Design review of the part built by this model. Coordinates are the model's own, in mm. A direction names the side the tool comes from. Coordinates: 2 decimals unless noted, no trailing zeros. Order: outer loops, then holes, each group sorted by start corner. A loop starts at its lowest first (then second) coordinate and runs counter-clockwise, first axis right, second up. Notation, with made-up numbers: (-9.75, 67.5) - (4.25, 67.5) arc R27 cw to (4.25, 104.5) - close; hole circle Ø1 at (-36.75, 42). An arc over 180 degrees is marked (long way). Write each question's results on one line, items separated by ' | '. Start each with the question number.
```python
from build123d import *
from OCP.BRepFilletAPI import BRepFilletAPI_MakeChamfer

# Parameters (mm, degrees)
BOSS_EXTRUDE1_DEPTH = 76.2
BOSS_EXTRUDE3_DEPTH = 152.4
SKETCH2_W           = 134.62
SKETCH2_H           = 39.37
CUT_EXTRUDE1_DEPTH  = 94.414090077
CHAMFER1_SIZE       = 2.54
SKETCH5_W           = 7.62
SKETCH5_H           = 6.35
BOSS_EXTRUDE4_DEPTH = 8.89
SKETCH6_W           = 134.62
SKETCH6_H           = 7.62
CUT_EXTRUDE2_DEPTH  = 95.091487925
FILLET1_R           = 2.54
FILLET2_R           = 1.27
CHAMFER2_SIZE       = 1.651
CHAMFER2_SIZE2      = 2.963635699


with BuildPart() as part:
    # Sketch1 → Boss-Extrude1 (new, symmetric)
    with BuildSketch(Plane(origin=(0, 0, 0), x_dir=(0, 0, -1), z_dir=(1, 0, 0))):
        Polygon((0, 0), (0, 12.7), (-9.525, 12.7), (-9.525, -50.8), (8.89, -50.8), (8.89, 0), align=None)
    extrude(amount=BOSS_EXTRUDE1_DEPTH, both=True)

    # Sketch4 → Boss-Extrude3 (add)
    with BuildSketch(Plane(origin=(76.2, 0, 0), x_dir=(0, 0, -1), z_dir=(1, 0, 0))):
        Polygon((8.89, 0), (21.59, 0), (21.59, -6.35), (8.89, -11.43), align=None)
    extrude(amount=-BOSS_EXTRUDE3_DEPTH)

    # Sketch2 → Cut-Extrude1 (cut, through all)
    with BuildSketch(Plane(origin=(0, 0, -8.89), x_dir=(-1, 0, 0), z_dir=(0, 0, -1))):
        with Locations((0, -31.115)):
            Rectangle(SKETCH2_W, SKETCH2_H)
    extrude(amount=-CUT_EXTRUDE1_DEPTH, mode=Mode.SUBTRACT)

    # Chamfer1
    chamfer1_edges = [part.edges().sort_by_distance(p)[0] for p in [
        (76.2, 12.7, 4.7625),
        (-76.2, 12.7, 4.7625),
    ]]
    chamfer(chamfer1_edges, length=CHAMFER1_SIZE)

    # Sketch5 → Boss-Extrude4 (add)
    with BuildSketch(Plane(origin=(76.2, 0, 0), x_dir=(0, 0, -1), z_dir=(1, 0, 0))):
        with Locations((17.78, 3.175)):
            Rectangle(SKETCH5_W, SKETCH5_H)
    boss_extrude4 = extrude(amount=-BOSS_EXTRUDE4_DEPTH)

    # Mirror1: Boss-Extrude4 across plane
    add(boss_extrude4.mirror(Plane(origin=(0, 0, 0), x_dir=(0, 0, 1), z_dir=(1, 0, 0))))

    # Sketch6 → Cut-Extrude2 (cut, through all)
    with BuildSketch(Plane(origin=(0, 0, 0), x_dir=(1, 0, 0), z_dir=(0, 1, 0))):
        with Locations((0, 17.78)):
            Rectangle(SKETCH6_W, SKETCH6_H)
    extrude(amount=-CUT_EXTRUDE2_DEPTH, mode=Mode.SUBTRACT)

    # Fillet1
    fillet1_edges = [part.edges().sort_by_distance(p)[0] for p in [
        (-71.755, -11.43, -8.89),
        (71.755, -11.43, -8.89),
        (-67.31, -4.699, -13.97),
        (67.31, -4.699, -13.97),
    ]]
    fillet(fillet1_edges, radius=FILLET1_R)

    # Fillet2
    fillet2_edges = [part.edges().sort_by_distance(p)[0] for p in [
        (67.31, 0, -15.24),
        (-67.31, 0, -15.24),
        (71.755, 0, -13.97),
        (-71.755, 0, -13.97),
    ]]
    fillet(fillet2_edges, radius=FILLET2_R)

    # Chamfer2: one chamfer whose edges measure the first distance from different faces: ONE call of the kernel's chamfer builder (chamfer() names one face for all edges)
    chamfer2_edges_1 = [part.edges().sort_by_distance(p)[0] for p in [
        (-71.755, -6.35, -21.59),
    ]]
    chamfer2_side_1 = [part.faces().sort_by_distance(p)[0] for p in [
        (-71.755, 0, -21.59),
    ]]
    chamfer2_edges_2 = [part.edges().sort_by_distance(p)[0] for p in [
        (71.755, 6.35, -21.59),
        (-71.755, 6.35, -21.59),
    ]]
    chamfer2_edges_3 = [part.edges().sort_by_distance(p)[0] for p in [
        (71.755, -6.35, -21.59),
    ]]
    chamfer2_side_3 = [part.faces().sort_by_distance(p)[0] for p in [
        (71.755, 0, -21.59),
    ]]
    chamfer2 = BRepFilletAPI_MakeChamfer(part.part.solid().wrapped)
    for e in chamfer2_edges_1:
        chamfer2.Add(CHAMFER2_SIZE, CHAMFER2_SIZE2, e.wrapped, chamfer2_side_1[0].wrapped)  # the first distance lies on this face
    for e in chamfer2_edges_2:
        chamfer2.Add(CHAMFER2_SIZE, e.wrapped)
    for e in chamfer2_edges_3:
        chamfer2.Add(CHAMFER2_SIZE, CHAMFER2_SIZE2, e.wrapped, chamfer2_side_3[0].wrapped)  # the first distance lies on this face
    add(Compound.cast(chamfer2.Shape()), mode=Mode.REPLACE)


solid = part.part
```
(1) Take a section at A-A (y = -43). State the section outline as (x, z) points (3 decimals), plus the area to 3 significant figures.
(2) To check wall thickness, follow line 1 along X through (y, z) = (-25, -8); line 2 along Z through (x, y) = (69, -40) (3 decimals); line 3 along Z through (x, y) = (-28, -4.5) (3 decimals). State the ranges of each line that lie inside material, in increasing order. Write a range as [from, to].
(3) Take a section at C-C (z = 6). State the section outline as (x, y) points.
(4) Take a section at B-B (x = 15.5). State the section outline as (y, z) points (3 decimals).
(5) Tool access review of faces 1 (the face through (-72, 4, -13.97)), 2 (the face through (1.07, -10.3, -11.72)), 3 (the face through (72, -32, -8.89)), 4 (the face through (-67.31, 1, -19)), 5 (the face through (72, 6.35, -17)): name each direction out of +Z, -Z, +X, -X, +Y, -Y from which nothing blocks a thin tool from reaching the whole face with its end or side.
(6) Clearance check with flat-ended pins moving along their axes: pin 1 (10 mm diameter, centred on x = -72.5, y = -31, fed in from -Z); pin 2 (14 mm diameter, centred on x = 1, y = 5.5, fed in from -Z); pin 3 (10 mm diameter, centred on x = -18, z = -9, fed in from +Y); pin 4 (15.5 mm diameter, centred on x = -12.5, z = -6, fed in from +Y). State where each tip first meets the part, or that it passes through.
(7) Mouldability with a two-part tool opening along X and no side actions: class faces 6 (the face through (-71.693, -6.094, -20.195)), 7 (the face through (1, -11.43, 0)), 8 (the face through (76.2, -20, 1)), 9 (the face through (-67.31, -31, -1)) as +X half, -X half, draft (parallel to the pull), parting line (faces both ways), or undercut.
(8) Take a section at D-D (y = -1.5). State the section outline as (x, z) points (3 decimals).
Worked out:
1) outline: (-76.2, -8.89) - (-67.31, -8.89) - (-67.31, 9.525) - (-76.2, 9.525) - close; (67.31, -8.89) - (76.2, -8.89) - (76.2, 9.525) - (67.31, 9.525) - close | area: 327 mm^2
2) line 1: [-76.2, -67.31], [67.31, 76.2] | line 2: [-8.89, 9.525] | line 3: [-13.97, 9.525]
3) outline: (-76.2, -50.8) - (-67.31, -50.8) - (-67.31, -11.43) - (67.31, -11.43) - (67.31, -50.8) - (76.2, -50.8) - (76.2, 10.16) - (73.66, 12.7) - (-73.66, 12.7) - (-76.2, 10.16) - close
4) outline: (-11.43, -8.89) - (-9.398, -13.97) - (0, -13.97) - (0, 0) - (12.7, 0) - (12.7, 9.525) - (-11.43, 9.525) - close
5) face 1: +X, -X, +Y | face 2: -Z, -Y | face 3: -Z, +X, -X, -Y | face 4: -Z, +Y | face 5: -Z, +X, -X, +Y
6) pin 1: z = -8.89 | pin 2: z = -13.97 | pin 3: y = 0 | pin 4: y = 12.7
7) face 6: draft | face 7: undercut | face 8: +X half | face 9: undercut
8) outline: (-76.2, -21.59) - (-67.31, -21.59) - (-67.31, -16.51) arc R2.54 cw to (-64.77, -13.97) - (64.77, -13.97) arc R2.54 cw to (67.31, -16.51) - (67.31, -21.59) - (76.2, -21.59) - (76.2, 9.525) - (-76.2, 9.525) - close
